Geometry check sheet. Reference: the model listing, model coordinates, mm. A direction names the side the tool comes from. Coordinates: 2 decimals unless noted, no trailing zeros. Order: outer loops, then holes, each group sorted by start corner. A loop starts at its lowest first (then second) coordinate and runs counter-clockwise, first axis right, second up. Notation, with made-up numbers: M 63,88.25 L 79,88.25 A21 ccw 79,119.25 Z; hole C 59.25,-34 d8. An arc over 180 degrees is marked long. One line per item, written item: value. Start each with the question number.
1) Sectioned sample at A-A, the plane z = 0. Enter the section's corners in (x, y).
2) Sectioned sample at C-C, the plane y = -26.5. Enter the section's corners in (x, z), then the cut area to 3 significant figures.
3) Draft check along X on faces 1 (the cylindrical face through (-6.883, -25.921, -30.996)), 2 (the flat face through (0, -27, 17.289)), 3 (the flat face through (0, -52.578, -21)). Enter one of: pulls with the +X half, pulls with the -X half, needs draft (parallel to the pull), parting line crosses it, or undercut.
4) Sectioned sample at B-B, the plane x = 0. Enter the section's corners in (y, z), then the cut area to 3 significant figures.
5) Access from +Z, -Z, +X, -X, +Y, -Y to the whole of each face (thin tool, end or side, straight path). Record for faces 4 (the flat face through (0, -27, -17.289)), 5 (the flat face through (0, 0, -21)).
6) Go/stop test with flat-tipped pins: P1, Ø1, axis at y = -10, z = 14.5, coming from the -X side; P2, Ø6, axis at y = -21, z = -20, coming from the -X side; P3, Ø2, axis at y = -37.5, z = -8.5, coming from the +X side. Record where each tip stops, or that it passes through.
7) Sectioned sample at D-D, the plane z = 23. Enter the section's corners in (x, y), then the cut area to 3 significant figures.
8) Thickness scan on L1, parallel to Z at x = 0, y = -23; L2, parallel to X at y = -9.5, z = 1.5; L3, parallel to Z at x = 4.5, y = -21. Record the ranges inside material, lowest first. Write a range as from..to.
```python
from build123d import *

# Parameters (mm, degrees)
F0_R     = 31.751454
F1_DEPTH = 52.578
F2_W     = 35.38131
F2_H     = 34.577188
F3_DEPTH = 141.478


with BuildPart() as f1:
    # F0 (on Front) → F1 (new body)
    with BuildSketch(Plane.XZ):
        Circle(F0_R)
    extrude(amount=F1_DEPTH)

    # F2 (on face) + F0 (on Front) → F3 (cut)
    with BuildSketch(Plane.XZ.offset(52.578)):
        Rectangle(F2_W, F2_H)
    with BuildSketch(Plane.XZ):
        Circle(F0_R)
    extrude(amount=-F3_DEPTH, mode=Mode.SUBTRACT)


solid = f1.part
```
Final values:
1. outline: M -31.75,-52.58 L -17.69,-52.58 L -17.69,0 L -31.75,0 Z; M 17.69,-52.58 L 31.75,-52.58 L 31.75,0 L 17.69,0 Z
2. outline: C 0,0 d63.5; hole M -17.69,-17.29 L 17.69,-17.29 L 17.69,17.29 L -17.69,17.29 Z
2. area: 1,940 mm^2
3. face 1: parting line crosses it
3. face 2: undercut
3. face 3: needs draft
4. outline: M -52.58,-31.75 L 0,-31.75 L 0,-17.29 L -52.58,-17.29 Z; M -52.58,17.29 L 0,17.29 L 0,31.75 L -52.58,31.75 Z
4. area: 1,520 mm^2
5. face 4: +Y, -Y
5. face 5: +Z, -Z, +X, -X, +Y
6. P1: stops at x = -28.5
6. P2: stops at x = -26.82
6. P3: stops at x = 30.85
7. outline: M -21.89,-52.58 L 21.89,-52.58 L 21.89,0 L -21.89,0 Z
7. area: 2,300 mm^2
8. L1: z = -31.75..-17.29, 17.29..31.75
8. L2: x = -31.72..-17.69, 17.69..31.72
8. L3: z = -31.43..-17.29, 17.29..31.43
